Can you work these out from the model? Positions are in its coordinate system, mm. A direction names the side the tool comes from. Give positions to 0.01 mm unless a question says otherwise; leave off trailing zeros. Write each loop counter-clockwise with the first axis right and the second up, starting at its lowest first coordinate (ties: lowest second). Pieces come first, ordered by that corner, then holes. Notation, with made-up numbers: (80, 21.5) -> (103, 21.5) arc R22 cw to (103, 46.5) -> close; hole circle Ø3 at (55.25, 7.5). An arc over 180 degrees is marked (long way). Answer as CSV lines item,"result". Start each with the question number.
1. I'm going to push flat-ended pins straight in: P1, Ø3, axis at y = -16.5, z = 5.5, coming from the +X side; P2, Ø3.5, axis at y = -1.5, z = 27, coming from the -X side; P3, Ø8, axis at x = 31.5, z = 22, coming from the +Y side. Where does each tip first touch, or does it pass through?
2. If we section it at B-B on x = 4: Write out the boundary of the cut face in (y, z) (3 decimals).
3. I need wall thicknesses on line 1 (Z direction, x = -27.5, y = 31) (3 decimals); line 2 (Y direction, x = -0.5, z = 10); line 3 (Y direction, x = -2.5, z = 33). Which ranges of each line are inside material? Lowest first, please. Write a range as [from, to].
4. If we mould it in two halves opening along X, with no side actions, what happens to faces 4 (the face through (-30.235, 23.183, 25.044)), 5 (the face through (-3.131, 5.525, 25)), 6 (the face through (7, 38, 50.8))? For each: pulls with the +X half, pulls with the -X half, needs draft (parallel to the pull), parting line crosses it, or undercut.
5. If we section it at C-C on z = 8: Write out the boundary of the cut face in (x, y), plus the area to 3 significant figures.
6. If we section it at D-D on x = -14: Write out the boundary of the cut face in (y, z) (3 decimals), plus the area to 3 significant figures.
7. On a 3-axis mill with a long thin cutter (end or side, diameter ignored), from which of +Z, -Z, +X, -X, +Y, -Y can I reach the whole of each face in a straight line? I mean faces 1 (the face through (3.131, -5.525, 25)), 2 (the face through (-11, 1, -3.175)), 3 (the face through (-7, 38, 0)). Say none if no direction works.
8. If we section it at A-A on y = 0: Write out the boundary of the cut face in (x, z) (3 decimals), plus the area to 3 significant figures.
Autodesk Inventor part; units mm, degrees
ref_plane "YZ Plane" through (0, 0, 0) normal (1, 0, 0) x (0, 1, 0)
ref_plane "XZ Plane" through (0, 0, 0) normal (0, 1, 0) x (-1, 0, 0)
ref_plane "XY Plane" through (0, 0, 0) normal (0, 0, 1) x (1, 0, 0)
sketch "Sketch1" plane through (0, 0, 0) normal (0, 0, 1) x (1, 0, 0)
  circle A0 centre (0, 0) radius 38.1
  dimension "d0" = 76.2
extrude "Extrusion1" add sketch "Sketch1" along normal blind 50.8
sketch "Sketch2" plane through (0, 0, 50.8) normal (0, 0, 1) x (1, 0, 0)
  circle A0 centre (0, 0) radius 50.8
  dimension "d3" = 101.6
extrude "Extrusion2" add sketch "Sketch2" along normal blind 3.175
sketch "Sketch3" plane through (0, 0, 0) normal (0, 0, -1) x (-1, 0, 0)
  circle A0 centre (0, 0) radius 50.8
extrude "Extrusion3" add sketch "Sketch3" along normal blind 3.175
sketch "Sketch4" plane through (0, 0, -3.175) normal (0, 0, -1) x (-1, 0, 0)
  line L0 (6.35, -3.6662) -> (0, -7.3323)
  line L1 (0, -7.3323) -> (-6.35, -3.6662)
  line L2 (-6.35, -3.6662) -> (-6.35, 3.6662)
  line L3 (-6.35, 3.6662) -> (0, 7.3323)
  line L4 (0, 7.3323) -> (6.35, 3.6662)
  line L5 (6.35, 3.6662) -> (6.35, -3.6662)
  point P0 (0, 0)
  point P1 (0, 0)
  dimension "d8" = 12.7
extrude "Extrusion4" cut sketch "Sketch4" against normal through all
properties part number "Spool" material "Aluminum 6061"
Computed values:
1,P1,"stops at x = 35.02"
1,P2,"stops at x = -38.1"
1,P3,"stops at y = 26.37"
2,outline,"(-50.642, -3.175) -> (-5.023, -3.175) -> (-5.023, 53.975) -> (-50.642, 53.975) -> (-50.642, 50.8) -> (-37.889, 50.8) -> (-37.889, 0) -> (-50.642, 0) -> close; (5.023, -3.175) -> (50.642, -3.175) -> (50.642, 0) -> (37.889, 0) -> (37.889, 50.8) -> (50.642, 50.8) -> (50.642, 53.975) -> (5.023, 53.975) -> close"
3,line 1,"z = [-3.175, 0], [50.8, 53.975]"
3,line 2,"y = [-38.1, -7.04], [7.04, 38.1]"
3,line 3,"y = [-38.02, -5.89], [5.89, 38.02]"
4,face 4,"parting line crosses it"
4,face 5,"undercut"
4,face 6,"needs draft"
5,outline,"circle Ø76.2 at (0, 0); hole (-6.35, -3.67) -> (0, -7.33) -> (6.35, -3.67) -> (6.35, 3.67) -> (0, 7.33) -> (-6.35, 3.67) -> close"
5,area,"4,420 mm2"
6,outline,"(-48.833, -3.175) -> (48.833, -3.175) -> (48.833, 0) -> (35.435, 0) -> (35.435, 50.8) -> (48.833, 50.8) -> (48.833, 53.975) -> (-48.833, 53.975) -> (-48.833, 50.8) -> (-35.435, 50.8) -> (-35.435, 0) -> (-48.833, 0) -> close"
6,area,"4,220 mm2"
7,face 1,"+Z, -Z"
7,face 2,"-Z, +X, -X, +Y, -Y"
7,face 3,"none"
8,outline,"(-50.8, -3.175) -> (-6.35, -3.175) -> (-6.35, 53.975) -> (-50.8, 53.975) -> (-50.8, 50.8) -> (-38.1, 50.8) -> (-38.1, 0) -> (-50.8, 0) -> close; (6.35, -3.175) -> (50.8, -3.175) -> (50.8, 0) -> (38.1, 0) -> (38.1, 50.8) -> (50.8, 50.8) -> (50.8, 53.975) -> (6.35, 53.975) -> close"
8,area,"3,790 mm2"
